For this review, take the finished solid that the model builds, in its own axes (mm). A direction names the side the tool comes from. Round coordinates to 2 decimals unless told otherwise and drop trailing zeros. Order: outer loops, then holes, each group sorted by start corner. A loop starts at its lowest first (then second) coordinate and runs counter-clockwise, first axis right, second up. Notation, with made-up numbers: (62, -38) - (108, -38) arc R21 ccw to (108, -4) - close; hole circle Ø3 at (59.25, 55.5). An arc over 180 degrees is marked (long way). One line per question, with ' | ' between items.
```python
from build123d import *

# Parameters (mm, degrees)
F3_R          = 9.8
F4_DEPTH      = 10
F4_DEPTH_BACK = 0.3
F6_R          = 15
F6_R_2        = 9.8
F7_DEPTH      = 1.5
F9_ANGLE      = 180
F10_R         = 6.5
F11_DEPTH     = 15


# Not quite as in the source:
# - a feature names something its author has since deleted; it is built from what else it names


with BuildPart() as f1:
    # F0 (on Top) → F1 (revolve)
    with BuildSketch(Plane.XY):
        with BuildLine():
            Line((0, 37), (0, -37))
            ThreePointArc((0, -37), (37, 0), (0, 37))
        make_face()
    revolve(axis=Axis((0, 0, 0), (0, -1, 0)))


with BuildPart() as f4:
    # F3 (on offset) → F4 (new body, two sides)
    with BuildSketch(Plane.XY.offset(40)) as f4_sk:
        Circle(F3_R)
    extrude(amount=-F4_DEPTH)
    extrude(f4_sk.sketch, amount=F4_DEPTH_BACK)

    # F5: cut F1
    add(f1.part, mode=Mode.SUBTRACT)

    # F6 (on face) → F7 (join)
    with BuildSketch(Plane.XY.offset(40.3)):
        Circle(F6_R)
        Circle(F6_R_2, mode=Mode.SUBTRACT)
        Circle(F6_R_2)
    extrude(amount=F7_DEPTH)


with BuildPart() as f4_1:
    # F9: moved
    add(f4.part.rotate(Axis((0, 0, 41.8), (0, 1, 0)), F9_ANGLE))

    # F10 (on face) → F11 (join)
    with BuildSketch(Plane(origin=(0, 0, 41.8), x_dir=(1, 0, 0), z_dir=(0, 0, -1))):
        Circle(F10_R)
    extrude(amount=F11_DEPTH)

    # F12 (on Front) → F14 (revolve)
    with BuildSketch(Plane.XZ):
        with BuildLine():
            Line((-6.5, 36.8), (-6.5, 41.8))
            Line((-6.5, 41.8), (-15, 41.8))
            add(Edge.make_bspline(
                [(-15, 41.8), (-14.5252337679, 40.5401661992), (-10.4554320312, 37.7730797784), (-8.2265594974, 37.2042804956), (-6.5, 36.8)],
                knots=[0, 0, 0, 0, 0.5265068143, 1, 1, 1, 1], degree=3))
        make_face()
    revolve(axis=Axis((0, 0, 37.5033216551), (0, 0, 1)))


solid = f4_1.part
```
(1) For probe 1 along X at (y, z) = (0, 29.25); probe 2 along Z at (x, y) = (-12, 3); probe 3 along Z at (x, y) = (-7, -13), list the stretches that pass through material, from the lowest coordinate up. Write a range as [from, to].
Output values:
probe 1: [-6.5, 6.5] | probe 2: [39.19, 43.3] | probe 3: [41.35, 43.3]
(2) Insertion check: pin 1 (5 mm diameter, centred on x = 3, z = 32, fed in from -Y); pin 2 (1.5 mm diameter, centred on x = -11, y = 0, fed in from -Z); pin 3 (6 mm diameter, centred on x = -7, y = -8.5, fed in from -Z). Each pin has a flat end and moves straight along its axis. Give the tip position at first contact, or say it passes through.
Output values:
pin 1: y = -6.48 | pin 2: z = 37.99 | pin 3: z = 37.17
(3) We need section A-A on z = 28.5. State the section outline as (x, y) points, plus the area to 3 significant figures.
Output values:
outline: circle Ø13 at (0, 0) | area: 133 mm^2
(4) For faces 1 (the flat face through (0, 0, 26.8)), 2 (the cylindrical face through (-5.158, 3.955, 31.87)), 3 (the flat face through (-3, -10, 43.3)), list the 3-axis set-ups (+Z, -Z, +X, -X, +Y, -Y) from which the entire face can be reached by the end or side of a thin tool; tool diameter is ignored.
Output values:
face 1: -Z, +X, -X, +Y, -Y | face 2: -Z | face 3: +Z
